The model under review builds one solid part; all positions refer to its coordinate system, in mm. Coordinates: 2 decimals unless noted, no trailing zeros. Write each loop counter-clockwise with the first axis right and the second up, starting at its lowest first coordinate (ties: lowest second). Pieces come first, ordered by that corner, then holes. Notation, with made-up numbers: (-16.75, 87) - (34.25, 87) arc R17 ccw to (34.25, 95) - close; hole circle Ø11 at (73.25, 54). An arc over 180 degrees is marked (long way). Use one line per item in the form item = value. Start each with the question number.
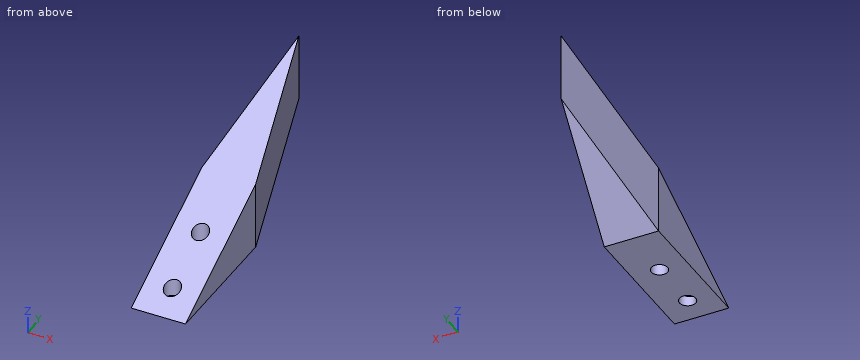
```python
from build123d import *

# Parameters (mm, degrees)
F1_DEPTH = 25
F3_DEPTH = 5.001
F4_DEPTH = 5.001
F5_R     = 1.5
F6_DEPTH = 25.001


with BuildPart() as f1:
    # F0 (on Top) → F1 (new body)
    with BuildSketch(Plane.XY):
        Polygon((-5, -25), (-5, -50), (5, -50), (5, -25), (0, 0), align=None)
    extrude(amount=F1_DEPTH)

    # F2 (on Right) → F3 (cut, through all)
    with BuildSketch(Plane.YZ):
        Polygon((-50, 0), (0, 25), (-50, 25), align=None)
        Polygon((-25, 0), (0, 0), (0, 12.5), align=None)
    extrude(amount=-F3_DEPTH, mode=Mode.SUBTRACT)

    # F3_face (on face) → F4 (cut, through all)
    with BuildSketch(Plane(origin=(0, -33.333333, 16.666667), x_dir=(0, 1, 0), z_dir=(-1, 0, 0))):
        Polygon((33.333333, -8.333333), (-16.666667, 16.666667), (-16.666667, -8.333333), align=None)
        Polygon((33.333333, 16.666667), (8.333333, 16.666667), (33.333333, 4.166667), align=None)
    extrude(amount=-F4_DEPTH, mode=Mode.SUBTRACT)

    # F5 (on face) → F6 (cut, through all)
    with BuildSketch(Plane(origin=(0, 0, 0), x_dir=(1, 0, 0), z_dir=(0, 0, -1))):
        with Locations((0, 35)):
            Circle(F5_R)
        with Locations((0, 45)):
            Circle(F5_R)
    extrude(amount=-F6_DEPTH, mode=Mode.SUBTRACT)


solid = f1.part
```
1. Take a section at C-C (y = -45). State the section outline as (x, z) points.
2. For P1, Ø2.5, axis at x = 0, y = -35, coming from the -Z side; P2, Ø1, axis at x = 1, y = -12, coming from the +Z side; P3, Ø1.5, axis at x = 1, y = -34, coming from the +Z side (3 decimals); P4, Ø12, axis at y = -17, z = 12, coming from the +X side, all flat-tipped, find the tip position at first contact; note any pin that passes through.
3. Take a section at D-D (x = -2). State the section outline as (y, z) points, plus the area to 3 significant figures.
4. Take a section at A-A (y = -35). State the section outline as (x, z) points, plus the area to 3 significant figures.
5. For L1, parallel to X at y = -35, z = 5; L2, parallel to Y at x = 0, z = 1.9; L3, parallel to Y at x = 0, z = 2.6, list the stretches that pass through material, from the lowest coordinate up.
6. Take a section at B-B (z = 4.25). State the section outline as (x, y) points.
Returned:
q1.outline = (-5, 0) - (-1.5, 0) - (-1.5, 2.5) - (-5, 2.5) - close; (1.5, 0) - (5, 0) - (5, 2.5) - (1.5, 2.5) - close
q2.P1 = through
q2.P2 = 19.25
q2.P3 = 8.375
q2.P4 = 4.6
q3.outline = (-50, 0) - (-25, 0) - (-10, 7.5) - (-10, 20) - close
q3.area = 344 mm²
q4.outline = (-5, 0) - (-1.5, 0) - (-1.5, 7.5) - (-5, 7.5) - close; (1.5, 0) - (5, 0) - (5, 7.5) - (1.5, 7.5) - close
q4.area = 52.5 mm²
q5.L1 = -5 to -1.5, 1.5 to 5
q5.L2 = -43.5 to -36.5, -33.5 to -21.2
q5.L3 = -43.5 to -36.5, -33.5 to -19.8
q6.outline = (-5, -41.5) - (5, -41.5) - (5, -25) - (3.3, -16.5) - (-3.3, -16.5) - (-5, -25) - close; hole circle Ø3 at (0, -35)
